Source: CAD feature listing. Evaluate the final solid. Frame: model axes, mm. A direction names the side the tool comes from. Round coordinates to 2 decimals unless told otherwise and drop trailing zeros. Write each loop counter-clockwise with the first axis right and the second up, starting at its lowest first coordinate (ties: lowest second). Pieces come first, ordered by that corner, then holes. Notation, with made-up numbers: M 57,-11.5 L 86,-11.5 A25 ccw 86,27.5 Z; hole C 87.5,-36.75 d10. An arc over 180 degrees is marked long. Use a Markdown table: item, result.
```python
from build123d import *

# Parameters (mm, degrees)
SKETCH1_W           = 82
SKETCH1_H           = 52
BOSS_EXTRUDE1_DEPTH = 2
FILLET1_R           = 2
CUT_EXTRUDE1_DEPTH  = 49.590122453
SKETCH3_R           = 2
CUT_EXTRUDE2_DEPTH  = 49.590122453
SKETCH4_R           = 3.5
SKETCH4_W           = 10
SKETCH4_H           = 14
SKETCH4_W_2         = 12.5
SKETCH4_H_2         = 11.25
CUT_EXTRUDE3_DEPTH  = 49.590122453


with BuildPart() as part:
    # Sketch1 → Boss-Extrude1 (new body)
    with BuildSketch(Plane.XY):
        Rectangle(SKETCH1_W, SKETCH1_H)
    extrude(amount=BOSS_EXTRUDE1_DEPTH)

    # Fillet1
    fillet1_edges = [part.edges().sort_by_distance(p)[0] for p in [
        (-41, 26, 1),
        (41, 26, 1),
        (41, -26, 1),
        (-41, -26, 1),
    ]]
    fillet(fillet1_edges, radius=FILLET1_R)

    # Sketch2 → Cut-Extrude1 (cut, through all)
    with BuildSketch(Plane.XY.offset(2)):
        with BuildLine():
            Line((-18.5, 20.5), (12.5, 20.5))
            ThreePointArc((12.5, 20.5), (14, 19), (12.5, 17.5))
            Line((12.5, 17.5), (-18.5, 17.5))
            ThreePointArc((-18.5, 17.5), (-20, 19), (-18.5, 20.5))
        make_face()
        with BuildLine():
            Line((-18.5, 15), (12.5, 15))
            ThreePointArc((12.5, 15), (14, 13.5), (12.5, 12))
            Line((12.5, 12), (-18.5, 12))
            ThreePointArc((-18.5, 12), (-20, 13.5), (-18.5, 15))
        make_face()
        with BuildLine():
            Line((-18.5, 9.5), (12.5, 9.5))
            ThreePointArc((12.5, 9.5), (14, 8), (12.5, 6.5))
            Line((12.5, 6.5), (-18.5, 6.5))
            ThreePointArc((-18.5, 6.5), (-20, 8), (-18.5, 9.5))
        make_face()
        with BuildLine():
            Line((-18.5, 4), (12.5, 4))
            ThreePointArc((12.5, 4), (14, 2.5), (12.5, 1))
            Line((12.5, 1), (-18.5, 1))
            ThreePointArc((-18.5, 1), (-20, 2.5), (-18.5, 4))
        make_face()
    extrude(amount=-CUT_EXTRUDE1_DEPTH, mode=Mode.SUBTRACT)

    # Sketch3 → Cut-Extrude2 (cut, through all)
    with BuildSketch(Plane.XY.offset(2)):
        with Locations((37.5, 22.5)):
            Circle(SKETCH3_R)
        with Locations((-37.5, 22.5)):
            Circle(SKETCH3_R)
        with Locations((37.5, -22.5)):
            Circle(SKETCH3_R)
        with Locations((-37.5, -22.5)):
            Circle(SKETCH3_R)
    extrude(amount=-CUT_EXTRUDE2_DEPTH, mode=Mode.SUBTRACT)

    # Sketch4 → Cut-Extrude3 (cut, through all)
    with BuildSketch(Plane.XY.offset(2)):
        with Locations((-31, -5.75)):
            Circle(SKETCH4_R)
        with Locations((-31, -16.25)):
            Circle(SKETCH4_R)
        with Locations((-36, 12)):
            Rectangle(SKETCH4_W, SKETCH4_H)
        with Locations((36, 12)):
            Rectangle(SKETCH4_W, SKETCH4_H)
        with Locations((27.5, -14.375)):
            Rectangle(SKETCH4_W_2, SKETCH4_H_2)
    extrude(amount=-CUT_EXTRUDE3_DEPTH, mode=Mode.SUBTRACT)


solid = part.part
```
Q1. Section B-B on x = 37.5. Return loops of the section in (y, z).
Results are:
| item | result |
|---|---|
| outline | M -26,0 L -24.5,0 L -24.5,2 L -26,2 Z; M -20.5,0 L 5,0 L 5,2 L -20.5,2 Z; M 19,0 L 20.5,0 L 20.5,2 L 19,2 Z; M 24.5,0 L 26,0 L 26,2 L 24.5,2 Z |
Q2. Reachability of faces 1 (the cylindrical face through (14, 2.5, 1)), 2 (the flat face through (41, -10, 1)), 3 (the flat face through (36, 5, 1)) from +Z, -Z, +X, -X, +Y, -Y: full face, straight path, thin tool, end or side. Return the list, or none.
Results are:
| item | result |
|---|---|
| face 1 | +Z, -Z |
| face 2 | +Z, -Z, +X, +Y, -Y |
| face 3 | +Z, -Z, +X |
Q3. Mould query, pull axis Y, two halves, no side actions, for faces 4 (the cylindrical face through (-27.767, -7.091, 1.014)), 5 (the cylindrical face through (40.43, 25.4, 1.01)), 6 (the flat face through (41, 21, 1)). Classes: +Y half, -Y half, draft (parallel to the pull), parting line (faces both ways), or undercut.
Results are:
| item | result |
|---|---|
| face 4 | undercut |
| face 5 | +Y half |
| face 6 | draft |
Q4. Line query: L1, parallel to Y at x = -2, z = 0.65; L2, parallel to Y at x = 37.5, z = 1.45; L3, parallel to Y at x = -29, z = 1.7. Output: solid intervals per line, ascending.
Results are:
| item | result |
|---|---|
| L1 | -26 to 1, 4 to 6.5, 9.5 to 12, 15 to 17.5, 20.5 to 26 |
| L2 | -26 to -24.5, -20.5 to 5, 19 to 20.5, 24.5 to 26 |
| L3 | -26 to -19.12, -13.38 to -8.62, -2.88 to 26 |
Q5. Section D-D on x = 3. Return loops of the section in (y, z).
Results are:
| item | result |
|---|---|
| outline | M -26,0 L 1,0 L 1,2 L -26,2 Z; M 4,0 L 6.5,0 L 6.5,2 L 4,2 Z; M 9.5,0 L 12,0 L 12,2 L 9.5,2 Z; M 15,0 L 17.5,0 L 17.5,2 L 15,2 Z; M 20.5,0 L 26,0 L 26,2 L 20.5,2 Z |
Q6. Section A-A on y = 22.5. Return loops of the section in (x, z).
Results are:
| item | result |
|---|---|
| outline | M -41,0 L -39.5,0 L -39.5,2 L -41,2 Z; M -35.5,0 L 35.5,0 L 35.5,2 L -35.5,2 Z; M 39.5,0 L 41,0 L 41,2 L 39.5,2 Z |
Q7. Section C-C on y = -5.75. Return loops of the section in (x, z), plus the area to 3 significant figures.
Results are:
| item | result |
|---|---|
| outline | M -41,0 L -34.5,0 L -34.5,2 L -41,2 Z; M -27.5,0 L 41,0 L 41,2 L -27.5,2 Z |
| area | 150 mm^2 |
